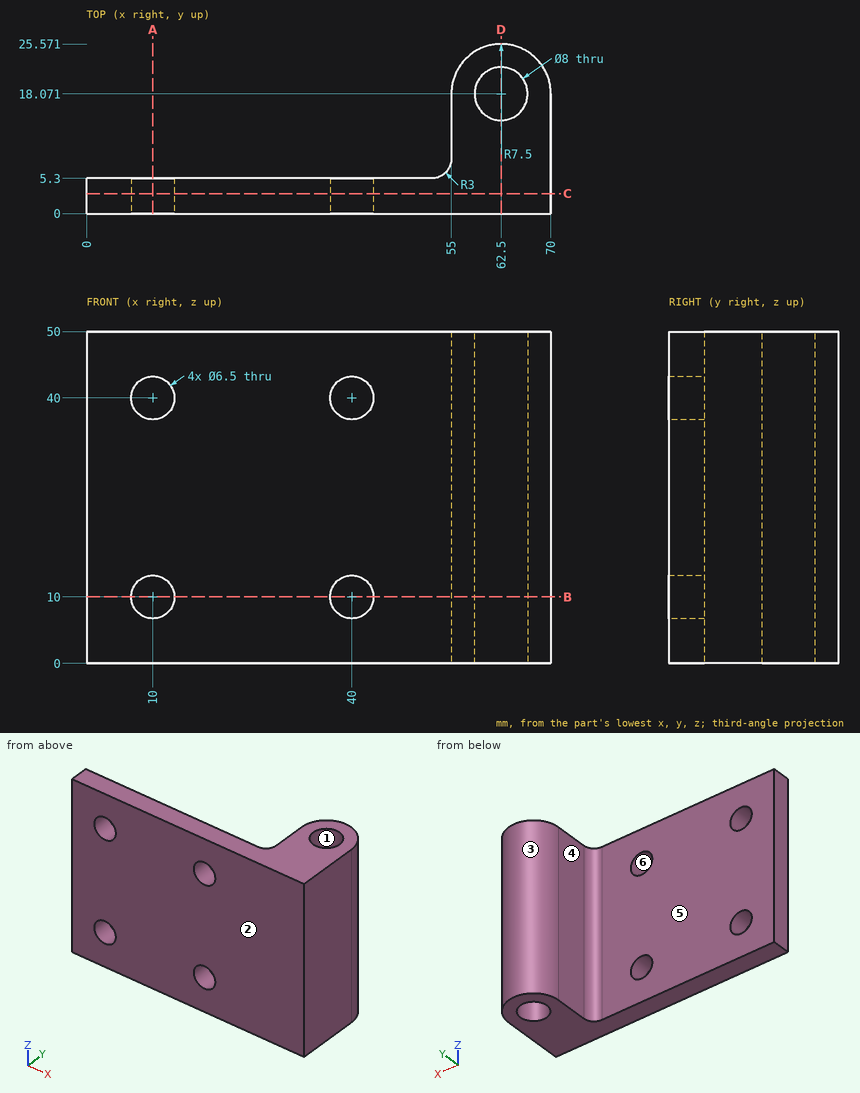
Study the drawing (mm; zero at the part's minimum x, y, z) and answer. A direction names the side the tool comes from. Round coordinates to 2 decimals unless told otherwise and drop trailing zeros. Write each loop counter-clockwise with the first axis right and the second up, starting at its lowest first coordinate (ties: lowest second). Pieces come first, ordered by that corner, then holes.
1) A cutting plane is placed at B-B (z = 10). Give the vertices of the cut face in (x, y), plus the area to 3 significant figures.
2) A cutting plane is placed at C-C (y = 3). Give the vertices of the cut face in (x, z), plus the area to 3 significant figures.
3) The mould has two halves that part along Y. Classify the marked faces 1, 2, 3 and 4: pulls with the +Y half, pulls with the -Y half, needs draft (parallel to the pull), parting line crosses it, or undercut.
4) Straight lines are drawn through the part: line 1 (X direction, y = 3.9, z = 10); line 2 (Y direction, x = 9, z = 29.5); line 3 (X direction, y = 10, z = 22). For each, find the intervals that lie inside material, in ascending order.
5) A tool of negligible diameter and unlimited length cuts with its end or side. For the marked faces 5 and 6, from which of +Z, -Z, +X, -X, +Y, -Y can it reach the whole face along a straight path? Write none if from no direction.
6) A cutting plane is placed at A-A (x = 10). Give the vertices of the cut face in (y, z), plus the area to 3 significant figures.
7) A cutting plane is placed at D-D (x = 62.5). Give the vertices of the cut face in (y, z).
8) Given pin 1 Ø5 at (x, z) = (10, 10) entering from -Y; pin 2 Ø10.5 at (y, z) = (12, 32) entering from -X; pin 3 Ø6 at (x, z) = (49, 22.5) entering from +Y; pin 4 Ø2 at (x, z) = (56, 19.5) entering from +Y, each flat-ended and moving along its own axis, determine where each tip first touches the part or whether it passes through.
Completed:
1. outline: (0, 0) - (6.75, 0) - (6.75, 5.3) - (0, 5.3) - close; (13.25, 0) - (36.75, 0) - (36.75, 5.3) - (13.25, 5.3) - close; (43.25, 0) - (70, 0) - (70, 18.07) arc R7.5 ccw to (55, 18.07) - (55, 8.3) arc R3 cw to (52, 5.3) - (43.25, 5.3) - close; hole circle Ø8 at (62.5, 18.07)
1. area: 534 mm2
2. outline: (0, 0) - (70, 0) - (70, 50) - (0, 50) - close; hole circle Ø6.5 at (10, 10); hole circle Ø6.5 at (10, 40); hole circle Ø6.5 at (40, 10); hole circle Ø6.5 at (40, 40)
2. area: 3,370 mm2
3. face 1: undercut
3. face 2: pulls with the -Y half
3. face 3: pulls with the +Y half
3. face 4: needs draft
4. line 1: x = 0 to 6.75, 13.25 to 36.75, 43.25 to 70
4. line 2: y = 0 to 5.3
4. line 3: x = 55 to 70
5. face 5: +Z, -Z, -X, +Y
5. face 6: +Y, -Y
6. outline: (0, 0) - (5.3, 0) - (5.3, 6.75) - (0, 6.75) - close; (0, 13.25) - (5.3, 13.25) - (5.3, 36.75) - (0, 36.75) - close; (0, 43.25) - (5.3, 43.25) - (5.3, 50) - (0, 50) - close
6. area: 196 mm2
7. outline: (0, 0) - (14.07, 0) - (14.07, 50) - (0, 50) - close; (22.07, 0) - (25.57, 0) - (25.57, 50) - (22.07, 50) - close
8. pin 1: passes through
8. pin 2: stops at x = 54.57
8. pin 3: stops at y = 5.3
8. pin 4: stops at y = 23.17
